The figure shows three views and two pictorial views of one solid part (mm, origin at its lowest corner). Answer the questions. Give positions to 0.01 mm unless a question says otherwise; leave off trailing zeros. Order: outer loops, then holes, each group sorted by start corner. A loop starts at its lowest first (then second) coordinate and runs counter-clockwise, first axis right, second up. Notation, with made-up numbers: (27, -24) -> (55, -24) arc R17 ccw to (55, 9) -> close; hole circle Ø11 at (-7.75, 28). An arc over 180 degrees is marked (long way). Use one line per item in the form item = value.
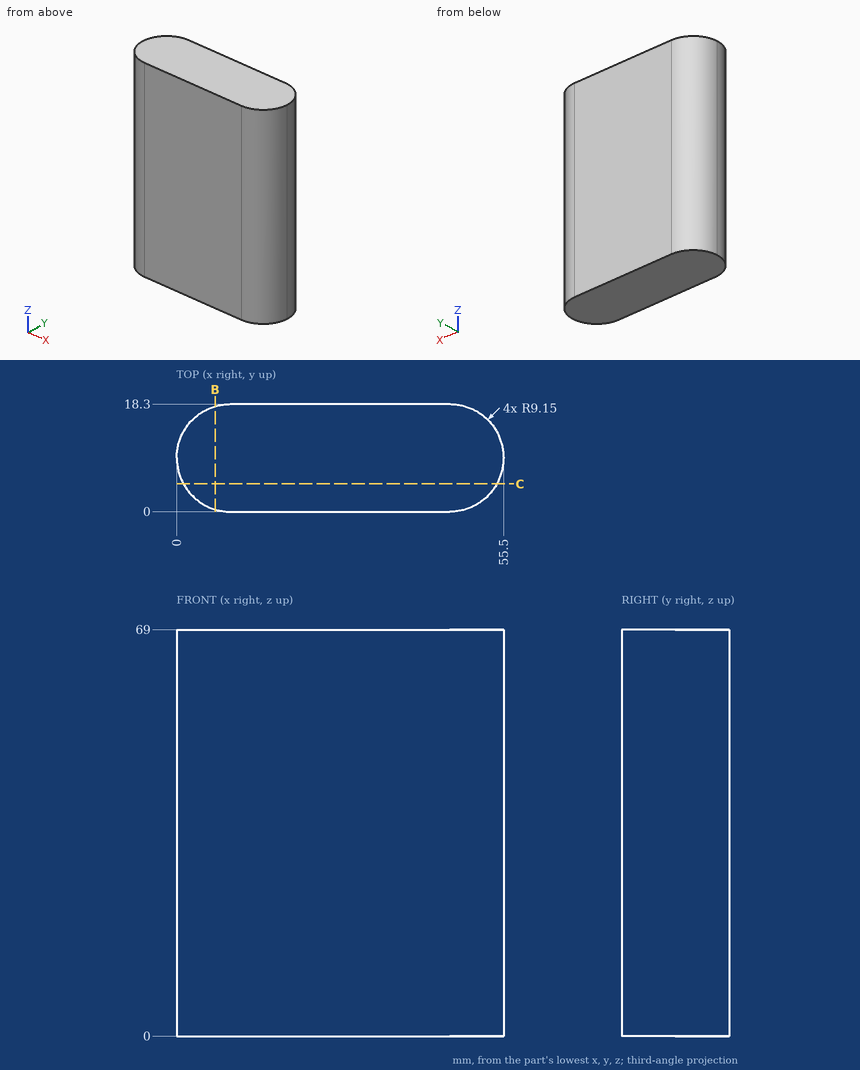
Item 1: The part is cut by section C-C on y = 4.75. Give the vertices of the cut face in (x, z).
Checks:
outline = (1.13, 0) -> (54.37, 0) -> (54.37, 69) -> (1.13, 69) -> close
Item 2: Straight lines are drawn through the part: L1, parallel to X at y = 17.5, z = 59; L2, parallel to X at y = 4, z = 12.5; L3, parallel to Y at x = 50, z = 19. For each, find the intervals that lie inside material, in ascending order. Write a range as from..to.
Checks:
L1 = 5.41..50.09
L2 = 1.59..53.91
L3 = 0.76..17.54
Item 3: The part is cut by section B-B on x = 6.5. Give the vertices of the cut face in (y, z), and give its area (3 significant figures).
Checks:
outline = (0.39, 0) -> (17.91, 0) -> (17.91, 69) -> (0.39, 69) -> close
area = 1,210 mm²
Item 4: Given pin 1 Ø6 at (y, z) = (10, 16) entering from -X; pin 2 Ø6 at (y, z) = (3.5, 13.5) entering from +X; pin 3 Ø1.5 at (y, z) = (4.5, 38) entering from +X, each flat-ended and moving along its own axis, determine where each tip first touches the part or whether it passes through.
Checks:
pin_1 = 0
pin_2 = 55.11
pin_3 = 54.63
